Part print with two shaded views. Sizes in mm from the minimum x, y, z corner. Round coordinates to 2 decimals unless told otherwise and drop trailing zeros. Write each loop counter-clockwise with the first axis right and the second up, starting at its lowest first coordinate (ties: lowest second). Pieces come first, ordered by that corner, then holes. Notation, with made-up numbers: (-24, -12) -> (-3, -12) arc R25 ccw to (-3, 22) -> close; hole circle Ø7 at (59, 82.5). An arc over 180 degrees is marked (long way). Answer in a Markdown table with one row per item.
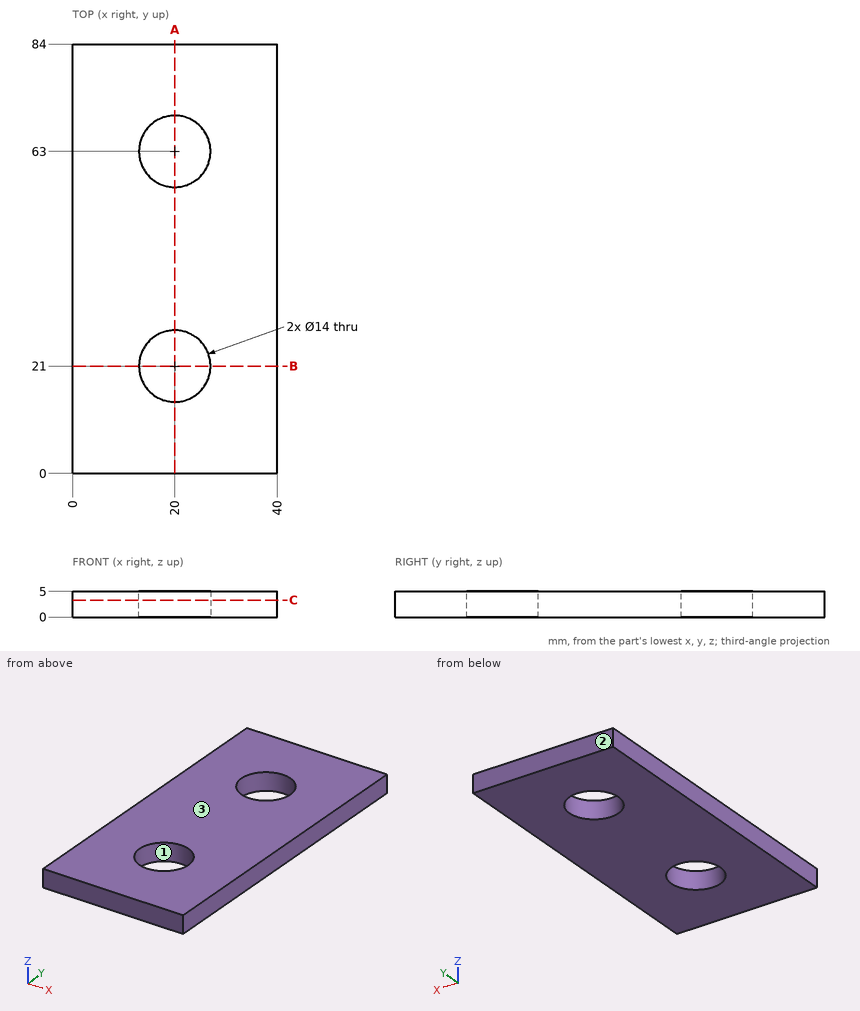
Q1. Saw through at B-B on y = 21. Write the cut outline in (x, z), plus the area to 3 significant figures.
A:
| item | result |
|---|---|
| outline | (0, 0) -> (13, 0) -> (13, 5) -> (0, 5) -> close; (27, 0) -> (40, 0) -> (40, 5) -> (27, 5) -> close |
| area | 130 mm² |
Q2. Saw through at A-A on x = 20. Write the cut outline in (y, z), plus the area to 3 significant figures.
A:
| item | result |
|---|---|
| outline | (0, 0) -> (14, 0) -> (14, 5) -> (0, 5) -> close; (28, 0) -> (56, 0) -> (56, 5) -> (28, 5) -> close; (70, 0) -> (84, 0) -> (84, 5) -> (70, 5) -> close |
| area | 280 mm² |
Q3. Saw through at C-C on z = 3.3. Write the cut outline in (x, y).
A:
| item | result |
|---|---|
| outline | (0, 0) -> (40, 0) -> (40, 84) -> (0, 84) -> close; hole circle Ø14 at (20, 21); hole circle Ø14 at (20, 63) |
Q4. Wall check: line 1 (Y direction, x = 20.5, z = 2.8); line 2 (Y direction, x = 16, z = 2.4); line 3 (X direction, y = 16, z = 4.2). Give the ranges that are in metal, low to high. Write a range as [from, to].
A:
| item | result |
|---|---|
| line 1 | [0, 14.02], [27.98, 56.02], [69.98, 84] |
| line 2 | [0, 15.26], [26.74, 57.26], [68.74, 84] |
| line 3 | [0, 15.1], [24.9, 40] |
Q5. Two-plate mould, pull along Y, no slides. Class the marked faces 1, 2 and 3: released by +Y, released by -Y, zero draft, split by the parting line, or undercut.
A:
| item | result |
|---|---|
| face 1 | undercut |
| face 2 | released by +Y |
| face 3 | zero draft |
